```python
from build123d import *

# Parameters (mm, degrees)
SKETCH001_R     = 4
POCKET_DEPTH    = 110
POCKET001_DEPTH = 45
CHAMFER_SIZE    = 1


with BuildPart() as part:
    # Sketch → Revolution (revolve)
    with BuildSketch(Plane.XY):
        Polygon((0, 0), (0, 30), (110, 40), (110, 0), align=None)
    revolve(axis=Axis((0, 0, 0), (1, 0, 0)))

    # Sketch001 (on Face1 of Revolution) → Pocket (cut)
    with BuildSketch(Plane(origin=(0, 0, 0), x_dir=(0, -1, 0), z_dir=(-1, 0, 0))):
        Circle(SKETCH001_R)
    extrude(amount=-POCKET_DEPTH, mode=Mode.SUBTRACT)

    # Sketch002 (on Face4 of Pocket) → Pocket001 (cut)
    with BuildSketch(Plane.YZ.offset(110)):
        Polygon((3.897114, 6.75), (-3.897114, 6.75), (-7.794229, 0), (-3.897114, -6.75), (3.897114, -6.75), (7.794229, 0), align=None)
    extrude(amount=-POCKET001_DEPTH, mode=Mode.SUBTRACT)

    # Chamfer
    chamfer_edges = [part.edges().sort_by_distance(p)[0] for p in [
        (110, 0, -6.75),
        (110, 0, 6.75),
        (110, 5.845671, 3.375),
        (110, 5.845671, -3.375),
        (110, -5.845671, 3.375),
        (110, -5.845671, -3.375),
    ]]
    chamfer(chamfer_edges, length=CHAMFER_SIZE)


solid = part.part
```
CAD build for the part. Positions are in the model's coordinates, mm. A direction names the side the tool comes from. Give positions to 0.01 mm unless a question says otherwise; leave off trailing zeros. Write each loop counter-clockwise with the first axis right and the second up, starting at its lowest first coordinate (ties: lowest second). Pieces come first, ordered by that corner, then holes. Notation, with made-up numbers: (-23.75, -31) -> (2.25, -31) arc R32 cw to (2.25, -3) -> close; hole circle Ø8 at (1.5, 37.5). An arc over 180 degrees is marked (long way). Write each question's results on one line, items separated by ' | '.
1. Cut at C-C, the plane x = 88.5. Write the cut outline in (y, z).
Geometry check:
outline: circle Ø76.09 at (0, 0); hole (-7.79, 0) -> (-3.9, -6.75) -> (3.9, -6.75) -> (7.79, 0) -> (3.9, 6.75) -> (-3.9, 6.75) -> close
2. Which spindle directions (+Z, -Z, +X, -X, +Y, -Y) get a long thin tool onto all of the face, cutting with end or side? Do faces 4 (the flat face through (0, 0, -6)), 5 (the flat face through (87, 0, 6.75)). Say none if no direction does.
Geometry check:
face 4: +Z, -Z, -X, +Y, -Y | face 5: +X
3. Two-plate mould, pull along Z, no slides. Class faces 1 (the flat face through (109.493, -6.241, 3.676)), 2 (the flat face through (110, -1, -8)), 3 (the conical face through (55.77, 33.45, 10.53)): pulls with the +Z half, pulls with the -Z half, needs draft (parallel to the pull), parting line crosses it, or undercut.
Geometry check:
face 1: undercut | face 2: needs draft | face 3: parting line crosses it
4. Wall check: probe 1 along Z at (x, y) = (40, 0); probe 2 along Z at (x, y) = (49, 0); probe 3 along Y at (x, z) = (74.5, -4). Give the ranges that are in metal, low to high. Write a range as [from, to].
Geometry check:
probe 1: [-33.64, -4], [4, 33.64] | probe 2: [-34.45, -4], [4, 34.45] | probe 3: [-36.55, -5.48], [5.48, 36.55]
5. Cut at D-D, the plane x = 56. Write the cut outline in (y, z).
Geometry check:
outline: circle Ø70.18 at (0, 0); hole circle Ø8 at (0, 0)
6. Drop flat-ended pins along their axis: P1, Ø2.5, axis at x = 91.5, y = 1, coming from the +Z side; P2, Ø4, axis at x = 87.5, y = 1, coming from the -Z side; P3, Ø7, axis at y = -1.5, z = 1.5, coming from the +X side. Give the stop position or say it passes through.
Geometry check:
P1: z = 38.42 | P2: z = -38.13 | P3: x = 65
7. Cut at A-A, the plane y = 0. Write the cut outline in (x, z).
Geometry check:
outline: (0, -30) -> (110, -40) -> (110, -7.75) -> (109, -6.75) -> (65, -6.75) -> (65, -4) -> (0, -4) -> close; (0, 4) -> (65, 4) -> (65, 6.75) -> (109, 6.75) -> (110, 7.75) -> (110, 40) -> (0, 30) -> close
8. Cut at B-B, the plane x = 77. Write the cut outline in (y, z).
Geometry check:
outline: circle Ø74 at (0, 0); hole (-7.79, 0) -> (-3.9, -6.75) -> (3.9, -6.75) -> (7.79, 0) -> (3.9, 6.75) -> (-3.9, 6.75) -> close
